Build history of the part. All positions in model axes, mm. A direction names the side the tool comes from. Give positions to 0.01 mm unless a question says otherwise; leave off trailing zeros. Loops run counter-clockwise (first coordinate to the right, second up) from the corner with the lowest first, then second, coordinate; pieces in that order, holes last. Notation, with made-up numbers: (78.25, -8) - (97.25, -8) arc R24 ccw to (97.25, 4) - close; hole circle Ø1 at (29.5, 73.25). An arc over 180 degrees is marked (long way). Return JSON: item names as keys, results as strings. Group by question number.
1) Drill centre lines: probe 1 along X at (y, z) = (4.75, 5.5); probe 2 along X at (y, z) = (0.45, 0); probe 3 along Y at (x, z) = (-0.25, 3.75). Where is each one in solid material? Low to high. Write a range as from..to.
2) Slice it at D-D (z = -4). List the corners of the cut face in (x, y), and give its area (3 significant figures).
3) Slice it at A-A (y = 3.5). List the corners of the cut face in (x, z).
4) Slice it at B-B (z = 0). List the corners of the cut face in (x, y), and give its area (3 significant figures).
5) 3-axis set-ups, long thin cutter, end or side, ignore diameter. For faces 5 (the face through (0.9, 0.49, 2.86)), 6 (the face through (13, 6, 0)), 7 (the face through (-15, 6, 0)): which of +Z, -Z, +X, -X, +Y, -Y reach the whole face in a straight line?
6) Drop a flat-ended pin along its axis: pin 1 (4 mm diameter, centred on x = 5, z = -1, fed in from -Y). Give the stop position or say it passes through.
7) Mould opens along Z. For faces 1 (the face through (0.9, 11.59, 2.86)), 2 (the face through (15, 6, 0)), 3 (the face through (0, 11.2, 0)), 4 (the face through (-0.2, 11.2, 7)) say: released by +Z, released by -Z, zero draft, split by the parting line, or undercut.
8) Slice it at C-C (x = 0.5). List the corners of the cut face in (y, z).
```python
from build123d import *

# Parameters (mm, degrees)
SKETCH_1_W      = 30
SKETCH_1_H      = 14
SKETCH_1_R      = 3
EXTRUDE_1_DEPTH = 1
SKETCH_2_W      = 2
SKETCH_2_H      = 14
EXTRUDE_2_DEPTH = 10
SKETCH_3_W      = 30
SKETCH_3_H      = 14
SKETCH_3_R      = 3
EXTRUDE_3_DEPTH = 1
SKETCH_4_R      = 3
EXTRUDE_4_DEPTH = 0.2


with BuildPart() as part:
    # Эскиз1 → Бобышка-Вытянуть1 (new body)
    with BuildSketch(Plane(origin=(0, 0, 0), x_dir=(1, 0, 0), z_dir=(0, 1, 0))):
        Rectangle(SKETCH_1_W, SKETCH_1_H)
        with Locations(Location((0, 0, 0), (0, 0, 270))):
            Circle(SKETCH_1_R, mode=Mode.SUBTRACT)
    extrude(amount=EXTRUDE_1_DEPTH)

    # Эскиз2 → Бобышка-Вытянуть2 (add)
    with BuildSketch(Plane(origin=(0, 1, 0), x_dir=(1, 0, 0), z_dir=(0, 1, 0))):
        with Locations((-14, 0)):
            Rectangle(SKETCH_2_W, SKETCH_2_H)
        with Locations((14, 0)):
            Rectangle(SKETCH_2_W, SKETCH_2_H)
    extrude(amount=EXTRUDE_2_DEPTH)

    # Эскиз3 → Бобышка-Вытянуть3 (add)
    with BuildSketch(Plane(origin=(0, 11, 0), x_dir=(1, 0, 0), z_dir=(0, 1, 0))):
        Rectangle(SKETCH_3_W, SKETCH_3_H)
        with Locations(Location((0, 0, 0), (0, 0, 270))):
            Circle(SKETCH_3_R, mode=Mode.SUBTRACT)
    extrude(amount=EXTRUDE_3_DEPTH)

    # Эскиз4 → Бобышка-Вытянуть4 (add)
    with BuildSketch(Plane.XZ.offset(-11)):
        with Locations(Location((0, 0, 0), (0, 0, 270))):
            Circle(SKETCH_4_R)
    extrude(amount=-EXTRUDE_4_DEPTH)


solid = part.part
```
Results:
{
 "1": {"probe 1": "-15..-13, 13..15", "probe 2": "-15..-3, 3..15", "probe 3": "0..1, 11..12"},
 "2": {"outline": "(-15, 0) - (15, 0) - (15, 12) - (-15, 12) - close; hole (-13, 1) - (13, 1) - (13, 11) - (-13, 11) - close", "area": "100 mm2"},
 "3": {"outline": "(-15, -7) - (-13, -7) - (-13, 7) - (-15, 7) - close; (13, -7) - (15, -7) - (15, 7) - (13, 7) - close"},
 "4": {"outline": "(-15, 0) - (-3, 0) - (-3, 1) - (-13, 1) - (-13, 11) - (13, 11) - (13, 1) - (3, 1) - (3, 0) - (15, 0) - (15, 12) - (3, 12) - (3, 11.2) - (-3, 11.2) - (-3, 12) - (-15, 12) - close", "area": "89.2 mm2"},
 "5": {"face 5": "-Y", "face 6": "+Z, -Z", "face 7": "+Z, -Z, -X, +Y, -Y"},
 "6": {"pin 1": "y = 0"},
 "7": {"face 1": "undercut", "face 2": "zero draft", "face 3": "undercut", "face 4": "released by +Z"},
 "8": {"outline": "(0, -7) - (1, -7) - (1, -2.96) - (0, -2.96) - close; (0, 2.96) - (1, 2.96) - (1, 7) - (0, 7) - close; (11, -7) - (12, -7) - (12, -2.96) - (11.2, -2.96) - (11.2, 2.96) - (12, 2.96) - (12, 7) - (11, 7) - close"}
}
